Source: CAD feature listing. Evaluate the final solid. Frame: model axes, mm. A direction names the side the tool comes from. Round coordinates to 2 decimals unless told otherwise and drop trailing zeros. Order: outer loops, then holes, each group sorted by start corner. A loop starts at its lowest first (then second) coordinate and runs counter-clockwise, first axis right, second up. Notation, with made-up numbers: (25, 80) - (30, 80) arc R22 cw to (30, 113) - close; hole circle Ø2 at (-11.75, 81.25). An arc over 180 degrees is marked (long way). Use one line per item in the form item = value. Start each with the question number.
Q1. Cut plane A-A, the plane z = 382.5. Return the cut outline in (x, y) (3 decimals).
Q2. Draft query along Y for faces 3 (the flat face through (3.175, 13, 255)), 4 (the flat face through (38, 0, 255)), 5 (the flat face through (35, 2, 517.525)). Return one class per face: released by +Y, released by -Y, zero draft, split by the parting line, or undercut.
Q3. Cut plane B-B, the plane x = 44. Return the cut outline in (y, z) (3 decimals).
Q4. Pin query (flat end, axial travel): pin 1 Ø6 at (y, z) = (12.7, 117.87) entering from -X. Return the tip coordinate at first contact, or that it passes through.
Q5. Set-up query: faces 1 (the flat face through (38, 3.175, 255)), 2 (the flat face through (76.2, 13, 255)). Return all of +Z, -Z, +X, -X, +Y, -Y with unobstructed straight access to the full face (end or side cutting, diameter ignored); none if empty.
Q6. Ray query, line 1 (X direction, y = 13.25, z = 125) (3 decimals); line 2 (Y direction, x = 13.5, z = 58) (3 decimals). Return the intervals inside material, ascending. Write a range as [from, to].
from build123d import *

# Parameters (mm, degrees)
SKETCH1_W           = 76.2
SKETCH1_H           = 25.4
SKETCH1_W_2         = 69.85
SKETCH1_H_2         = 19.05
BOSS_EXTRUDE1_DEPTH = 517.525
SKETCH3_R           = 3.3782
CUT_EXTRUDE1_DEPTH  = 77.2


with BuildPart() as part:
    # Sketch1 → Boss-Extrude1 (new body)
    with BuildSketch(Plane.XY):
        with Locations((38.1, 12.7)):
            Rectangle(SKETCH1_W, SKETCH1_H)
        with Locations((38.1, 12.7)):
            Rectangle(SKETCH1_W_2, SKETCH1_H_2, mode=Mode.SUBTRACT)
    extrude(amount=BOSS_EXTRUDE1_DEPTH)

    # Sketch3 → Cut-Extrude1 (cut, through all)
    with BuildSketch(Plane(origin=(76.2, 0, 0), x_dir=(0, 0, -1), z_dir=(1, 0, 0))):
        with Locations((-508.3937, 12.7)):
            Circle(SKETCH3_R)
        with Locations((-399.6563, 12.7)):
            Circle(SKETCH3_R)
    cut_extrude1 = extrude(amount=-CUT_EXTRUDE1_DEPTH, mode=Mode.SUBTRACT)

    # Mirror1: Cut-Extrude1 across plane
    add(cut_extrude1.mirror(Plane(origin=(0, 0, 258.7625), x_dir=(1, 0, 0), z_dir=(0, 0, -1))), mode=Mode.SUBTRACT)


solid = part.part
Completed:
q1.outline = (0, 0) - (76.2, 0) - (76.2, 25.4) - (0, 25.4) - close; hole (3.175, 3.175) - (73.025, 3.175) - (73.025, 22.225) - (3.175, 22.225) - close
q2.face_3 = undercut
q2.face_4 = released by -Y
q2.face_5 = zero draft
q3.outline = (0, 0) - (3.175, 0) - (3.175, 517.525) - (0, 517.525) - close; (22.225, 0) - (25.4, 0) - (25.4, 517.525) - (22.225, 517.525) - close
q4.pin_1 = through
q5.face_1 = +Z, -Z
q5.face_2 = +Z, -Z, +X, +Y, -Y
q6.line_1 = [0, 3.175], [73.025, 76.2]
q6.line_2 = [0, 3.175], [22.225, 25.4]
